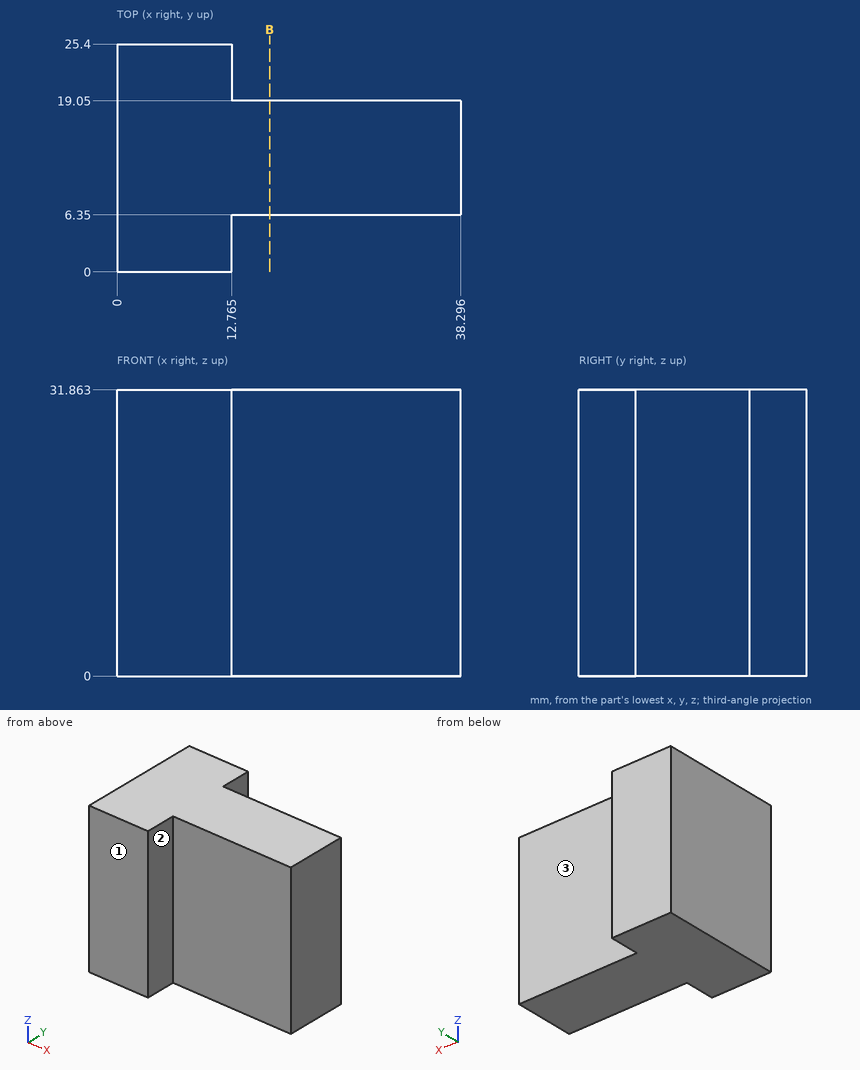
The drawing under review shows one solid part. Ordinate dimensions are in mm from its lowest x, y, z. A direction names the side the tool comes from. Round coordinates to 2 decimals unless told otherwise and drop trailing zeros. Loops run counter-clockwise (first coordinate to the right, second up) from the corner with the lowest first, then second, coordinate; pieces in that order, holes last. Notation, with made-up numbers: (56, 61) - (77, 61) arc R18 cw to (77, 73) - close; hole circle Ø5 at (27, 46). An arc over 180 degrees is marked (long way). Put each result on its own line as item: value. Start each with the question number.
1. Insertion check: P1, Ø5, axis at y = 1.5, z = 24, coming from the +X side (1 decimal); P2, Ø7.5, axis at x = 30, z = 14.5, coming from the +Y side; P3, Ø13, axis at x = 22, z = 16, coming from the -Y side. Each pin has a flat end and moves straight along its axis. Give the tip position at first contact, or say it passes through.
2. Consider section B-B on x = 17. State the section outline as (y, z) points, plus the area to 3 significant figures.
3. For the marked faces 1, 2 and 3, list the 3-axis set-ups (+Z, -Z, +X, -X, +Y, -Y) from which the entire face can be reached by the end or side of a thin tool; tool diameter is ignored.
4. For probe 1 along X at (y, z) = (20, 15) (1 decimal); probe 2 along Y at (x, z) = (32.5, 16), list the stretches that pass through material, from the lowest coordinate up. Write a range as [from, to].
Result sheet:
1. P1: x = 12.8
1. P2: y = 19.05
1. P3: y = 6.35
2. outline: (6.35, 0) - (19.05, 0) - (19.05, 31.86) - (6.35, 31.86) - close
2. area: 405 mm^2
3. face 1: +Z, -Z, +X, -X, -Y
3. face 2: +Z, -Z, +X, -Y
3. face 3: +Z, -Z, +X, +Y
4. probe 1: [0, 12.8]
4. probe 2: [6.35, 19.05]
